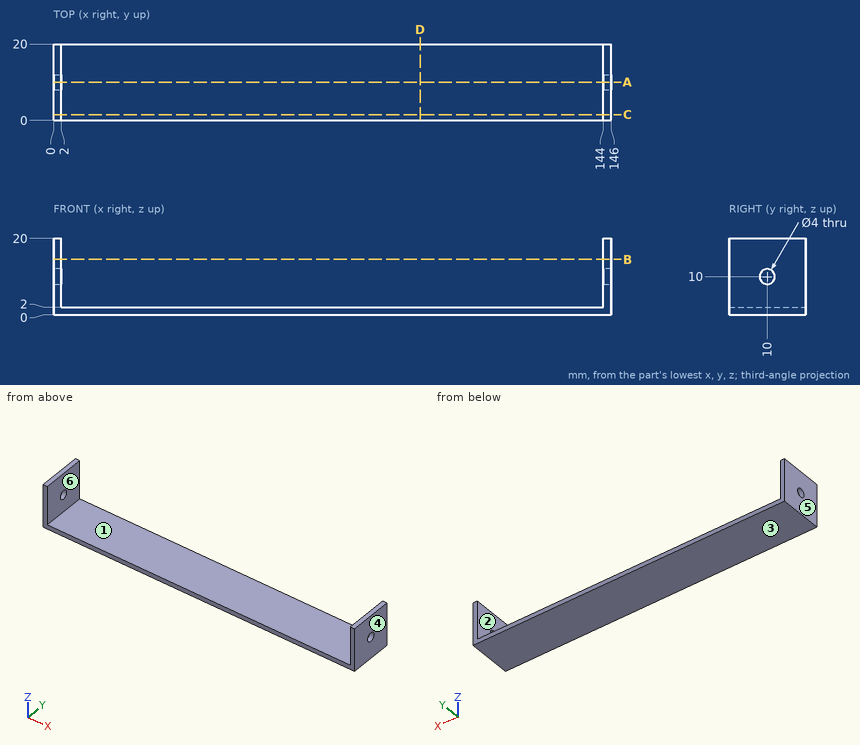
Geometry: see drawing. Coordinates: mm, zero at the bounding-box minimum. A direction names the side the tool comes from. Give positions to 0.01 mm unless a question says otherwise; leave off trailing zeros. Order: outer loops, then holes, each group sorted by start corner. A loop starts at its lowest first (then second) coordinate and runs counter-clockwise, first axis right, second up. Notation, with made-up numbers: (-38.75, -14) - (17.25, -14) arc R28 cw to (17.25, 10) - close; hole circle Ø11 at (-13.5, 61). An arc over 180 degrees is marked (long way). One line per item, written item: value.
1. Line query: probe 1 along Y at (x, z) = (1.25, 10); probe 2 along X at (y, z) = (2.5, 18.25). Output: solid intervals per line, ascending.
Determined:
probe 1: 0 to 8, 12 to 20
probe 2: 0 to 2, 144 to 146
2. Cut plane A-A, the plane y = 10. Output: boundary loops of the cut face in (x, z), and give its area (3 significant figures).
Determined:
outline: (0, 0) - (146, 0) - (146, 8) - (144, 8) - (144, 2) - (2, 2) - (2, 8) - (0, 8) - close; (0, 12) - (2, 12) - (2, 20) - (0, 20) - close; (144, 12) - (146, 12) - (146, 20) - (144, 20) - close
area: 348 mm2
3. Pin query (flat end, axial travel): pin 1 Ø5 at (x, y) = (109.5, 14.5) entering from +Z. Return the tip coordinate at first contact, or that it passes through.
Determined:
pin 1: z = 2
4. Draft query along X for the marked faces 1, 2, 3 and 4. Return one class per face: released by +X, released by -X, zero draft, split by the parting line, or undercut.
Determined:
face 1: undercut
face 2: undercut
face 3: zero draft
face 4: released by +X
5. Cut plane D-D, the plane x = 96. Output: boundary loops of the cut face in (y, z).
Determined:
outline: (0, 0) - (20, 0) - (20, 2) - (0, 2) - close
6. Reachability of the marked faces 5 and 6 from +Z, -Z, +X, -X, +Y, -Y: full face, straight path, thin tool, end or side. Return the list, or none.
Determined:
face 5: +Z, -Z, -X, +Y, -Y
face 6: +Z, +Y, -Y
7. Cut plane C-C, the plane y = 1.5. Output: boundary loops of the cut face in (x, z), and give its area (3 significant figures).
Determined:
outline: (0, 0) - (146, 0) - (146, 20) - (144, 20) - (144, 2) - (2, 2) - (2, 20) - (0, 20) - close
area: 364 mm2
8. Cut plane B-B, the plane z = 14.5. Output: boundary loops of the cut face in (x, y).
Determined:
outline: (0, 0) - (2, 0) - (2, 20) - (0, 20) - close; (144, 0) - (146, 0) - (146, 20) - (144, 20) - close
